from build123d import *

# Parameters (mm, degrees)
SKETCH1_R           = 5.5
SKETCH1_R_2         = 2.5
BOSS_EXTRUDE1_DEPTH = 4
SKETCH2_R           = 6.25
SKETCH2_R_2         = 2.5
BOSS_EXTRUDE2_DEPTH = 1
SKETCH3_R           = 4.7
SKETCH3_R_2         = 3.1
CUT_EXTRUDE1_DEPTH  = 0.25
CUT_EXTRUDE2_START  = -0.25
SKETCH4_R           = 4.7
SKETCH4_R_2         = 3.1
CUT_EXTRUDE2_DEPTH  = 0.25
CHAMFER1_SIZE       = 0.25


with BuildPart() as part:
    # Sketch1 → Boss-Extrude1 (new body)
    with BuildSketch(Plane(origin=(0, 0, 0), x_dir=(1, 0, 0), z_dir=(0, 1, 0))):
        with Locations(Location((0, 0, 0), (0, 0, 270))):
            Circle(SKETCH1_R)
        with Locations(Location((0, 0, 0), (0, 0, 270))):
            Circle(SKETCH1_R_2, mode=Mode.SUBTRACT)
    extrude(amount=BOSS_EXTRUDE1_DEPTH)

    # Sketch2 → Boss-Extrude2 (add)
    with BuildSketch(Plane(origin=(0, 4, 0), x_dir=(1, 0, 0), z_dir=(0, 1, 0))):
        with Locations(Location((0, 0, 0), (0, 0, 270))):
            Circle(SKETCH2_R)
        with Locations(Location((0, 0, 0), (0, 0, 270))):
            Circle(SKETCH2_R_2, mode=Mode.SUBTRACT)
    extrude(amount=BOSS_EXTRUDE2_DEPTH)

    # Sketch3 → Cut-Extrude1 (cut)
    with BuildSketch(Plane.XZ):
        with Locations(Location((0, 0, 0), (0, 0, 270))):
            Circle(SKETCH3_R)
        with Locations(Location((0, 0, 0), (0, 0, 270))):
            Circle(SKETCH3_R_2, mode=Mode.SUBTRACT)
    extrude(amount=-CUT_EXTRUDE1_DEPTH, mode=Mode.SUBTRACT)

    # Sketch4 → Cut-Extrude2 (cut)
    with BuildSketch(Plane(origin=(0, 5, 0), x_dir=(1, 0, 0), z_dir=(0, 1, 0)).offset(CUT_EXTRUDE2_START)):
        with Locations(Location((0, 0, 0), (0, 0, 90))):
            Circle(SKETCH4_R)
        with Locations(Location((0, 0, 0), (0, 0, 90))):
            Circle(SKETCH4_R_2, mode=Mode.SUBTRACT)
    extrude(amount=CUT_EXTRUDE2_DEPTH, mode=Mode.SUBTRACT)

    # Chamfer1
    chamfer1_edges = [part.edges().sort_by_distance(p)[0] for p in [
        (0, 5, -6.25),
    ]]
    chamfer(chamfer1_edges, length=CHAMFER1_SIZE)


solid = part.part
Source: CAD feature listing. Evaluate the final solid. Frame: model axes, mm. A direction names the side the tool comes from. Give positions to 0.01 mm unless a question says otherwise; leave off trailing zeros. Write each loop counter-clockwise with the first axis right and the second up, starting at its lowest first coordinate (ties: lowest second). Pieces come first, ordered by that corner, then holes. Notation, with made-up numbers: M -14.75,-7.5 L 40.25,-7.5 A36 ccw 40.25,29.5 Z; hole C 21,59.5 d4. An arc over 180 degrees is marked long. Return JSON: item names as keys, results as strings. Group by question number.
1) Set-up query: faces 1 (the face through (-2.44, 2.46, -0.54)), 2 (the face through (-5.37, 1.97, -1.19)), 3 (the face through (3.1, 4.75, -1)). Return all of +Z, -Z, +X, -X, +Y, -Y with unobstructed straight access to the full face (end or side cutting, diameter ignored); none if empty.
2) Material intervals for line 1 along X through (y, z) = (2.9, 0); line 2 along Y through (x, z) = (-1.25, 5.5); line 3 along Y through (x, z) = (-2.25, -3.5), sorted ascending. Write a range as [from, to].
3) Pull-direction query (X, two-part tool) for faces 4 (the face through (-3, 5, -4)), 5 (the face through (-3.1, 0.25, -1)), 6 (the face through (1.88, 4.37, 5.96)); classes: pulls with the +X half, pulls with the -X half, needs draft (parallel to the pull), parting line crosses it, or undercut.
4) Cut plane C-C, the plane y = 3.75. Output: boundary loops of the cut face in (x, z).
5) Pin query (flat end, axial travel): P1, Ø1, axis at y = 0.5, z = 2, coming from the -X side. Return the tip coordinate at first contact, or that it passes through.
Recorded:
{
 "1": {"face 1": "+Y, -Y", "face 2": "-Y", "face 3": "+Y"},
 "2": {"line 1": "x = [-5.5, -2.5], [2.5, 5.5]", "line 2": "y = [4, 5]", "line 3": "y = [0.25, 4.75]"},
 "3": {"face 4": "needs draft", "face 5": "undercut", "face 6": "parting line crosses it"},
 "4": {"outline": "C 0,0 d11; hole C 0,0 d5"},
 "5": {"P1": "stops at x = -5.29"}
}
